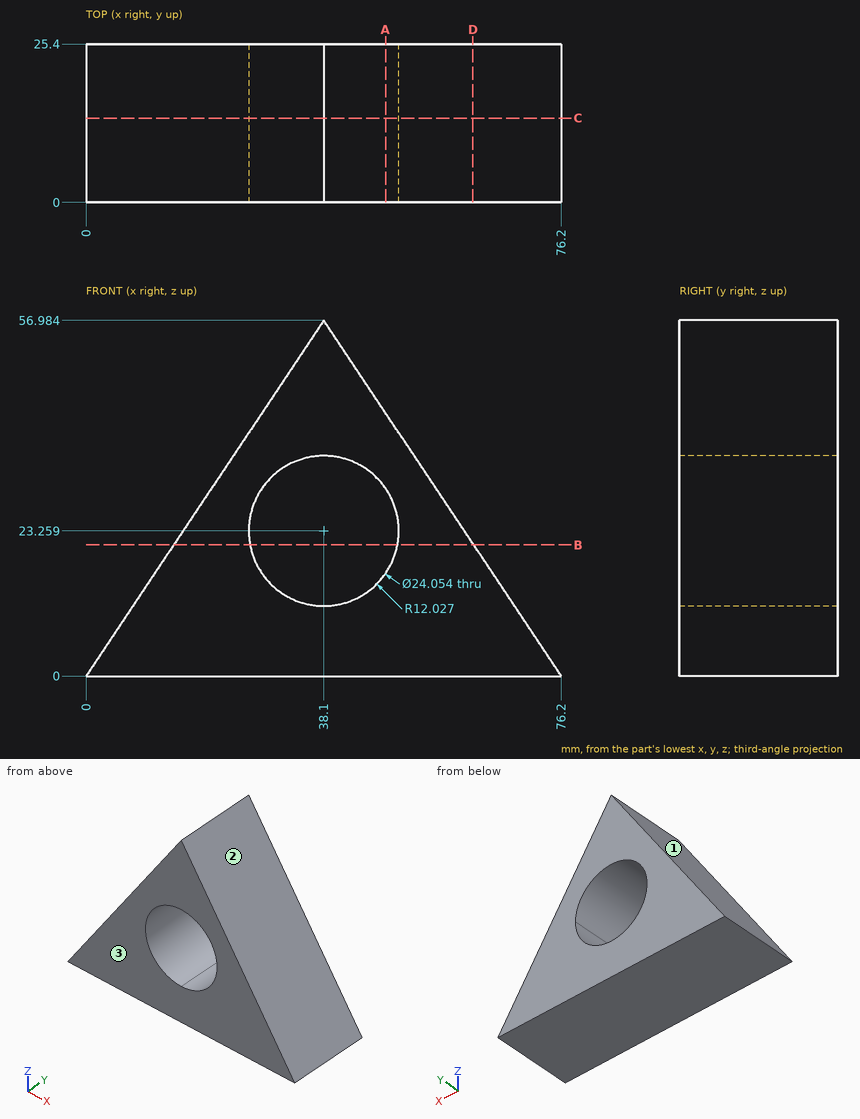
Verification items for this drawing (mm, ordinates from the low corner). Give positions to 0.01 mm unless a question says otherwise; leave off trailing zeros. Loops run counter-clockwise (first coordinate to the right, second up) from the corner with the lowest first, then second, coordinate; pieces in that order, holes last. Notation, with made-up numbers: (-11, -36) - (43, -36) arc R16 cw to (43, -10) - close; hole circle Ø4 at (40, -39). An arc over 180 degrees is marked (long way). Write item = value, one per line. Start each with the question number.
Q1. Cross-section at C-C, the plane y = 13.5. Enter the section's corners in (x, z) (1 decimal).
Q2. Cross-section at A-A, the plane x = 48. Enter the section's corners in (y, z), and give its area (3 significant figures).
Q3. Cross-section at B-B, the plane z = 21. Enter the section's corners in (x, y).
Q4. Thickness scan on line 1 (X direction, y = 17.25, z = 26) (1 decimal); line 2 (X direction, y = 20.25, z = 31.5); line 3 (Z direction, x = 8.5, y = 12) (1 decimal). Record the ranges inside material, lowest first.
Q5. Mould release check, pull along X, two halves, no side actions. Record for the marked faces 1, 2 and 3: released by +X, released by -X, zero draft, split by the parting line, or undercut.
Q6. Cross-section at D-D, the plane x = 62. Enter the section's corners in (y, z).
Q7. Depth check by flat-ended pin: P1, Ø3, axis at y = 19.5, z = 19, coming from the +X side; P2, Ø1.5, axis at y = 7, z = 18.5, coming from the +X side; P3, Ø5, axis at y = 8, z = 27, coming from the -X side. Enter the tip coordinate at first touch or a pass-through.
Answer key:
q1.outline = (0, 0) - (76.2, 0) - (38.1, 57) - close; hole circle Ø24.1 at (38.1, 23.3)
q2.outline = (0, 0) - (25.4, 0) - (25.4, 16.43) - (0, 16.43) - close; (0, 30.09) - (25.4, 30.09) - (25.4, 42.18) - (0, 42.18) - close
q2.area = 724 mm^2
q3.outline = (14.04, 0) - (26.29, 0) - (26.29, 25.4) - (14.04, 25.4) - close; (49.91, 0) - (62.16, 0) - (62.16, 25.4) - (49.91, 25.4) - close
q4.line_1 = 17.4 to 26.4, 49.8 to 58.8
q4.line_2 = 21.06 to 29.34, 46.86 to 55.14
q4.line_3 = 0 to 12.7
q5.face_1 = released by -X
q5.face_2 = released by +X
q5.face_3 = zero draft
q6.outline = (0, 0) - (25.4, 0) - (25.4, 21.24) - (0, 21.24) - close
q7.P1 = 64.5
q7.P2 = 64.33
q7.P3 = 16.38
